For this review, take the finished solid that the model builds, in its own axes (mm). Face numbers are marked on the shaded views. A direction names the side the tool comes from. Round coordinates to 2 decimals unless told otherwise and drop trailing zeros. Order: outer loops, then holes, each group sorted by start corner. A loop starts at its lowest first (then second) coordinate and runs counter-clockwise, first axis right, second up. Notation, with made-up numbers: M 37,15 L 62,15 A30 cw 62,45 Z; hole C 56,13 d7. An arc over 180 degrees is marked long. Write item = value, one per line. Start each with the question number.
from build123d import *

# Parameters (mm, degrees)
SKETCH_1_R          = 7
SKETCH_1_R_2        = 3.45
EXTRUDE_1_DEPTH     = 10
SKETCH_2_R          = 8.05
SKETCH_2_R_2        = 4
CUT_EXTRUDE_1_DEPTH = 8


with BuildPart() as part:
    # 草图1 → 凸台-拉伸1 (new body)
    with BuildSketch(Plane.XY):
        Polygon((-25, 0), (25, 0), (25, 26), (13, 85), (-13, 85), (-25, 26), align=None)
        with Locations((0, 73)):
            Circle(SKETCH_1_R, mode=Mode.SUBTRACT)
        with Locations((-15, 13)):
            Circle(SKETCH_1_R_2, mode=Mode.SUBTRACT)
        with Locations((15, 13)):
            Circle(SKETCH_1_R_2, mode=Mode.SUBTRACT)
    extrude(amount=EXTRUDE_1_DEPTH)

    # 草图2 → 切除-拉伸1 (cut)
    with BuildSketch(Plane(origin=(0, 0, 0), x_dir=(-1, 0, 0), z_dir=(0, 0, -1))):
        with Locations((0, 73)):
            Circle(SKETCH_2_R)
        with Locations((0, 73)):
            Circle(SKETCH_2_R_2, mode=Mode.SUBTRACT)
    extrude(amount=-CUT_EXTRUDE_1_DEPTH, mode=Mode.SUBTRACT)


solid = part.part
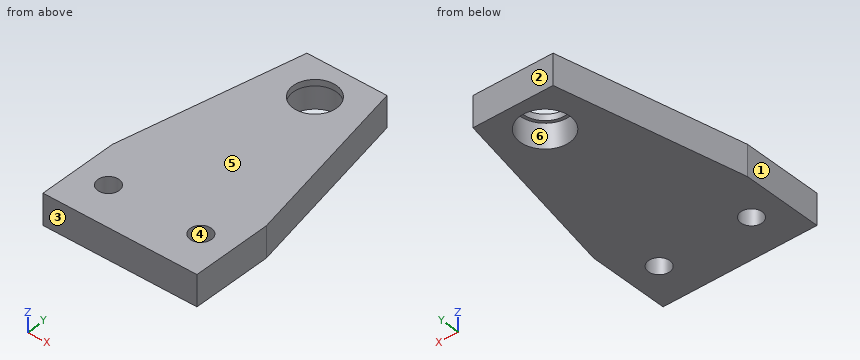
(1) We need section D-D, the plane y = 73. Write out the cut boundary in (x, z).
(2) We need section C-C, the plane z = 4.75. Write out the cut boundary in (x, y), then the cut area to 3 significant figures.
(3) For line 1 along Y through (x, z) = (0.5, 8.25); line 2 along Y through (x, z) = (0, 3); line 3 along X through (y, z) = (73, 9.1), list the stretches that pass through material, from the lowest coordinate up.
(4) We need section A-A, the plane x = 0. Write out the cut boundary in (y, z).
(5) We need section B-B, the plane y = 13. Write out the cut boundary in (x, z).
(6) Draft analysis for pull direction Y (two halves, no side actions). For the marked faces 1, 2, 3 and 4, state which applies: released by +Y, released by -Y, zero draft, split by the parting line, or undercut.
(7) Insertion check: pin 1 (1 mm diameter, centred on y = 51, z = 1, fed in from +X); pin 2 (4 mm diameter, centred on x = -15, y = 13, fed in from +Z); pin 3 (4 mm diameter, centred on y = 37, z = 5.5, fed in from +X); pin 4 (3 mm diameter, centred on y = 32.5, z = 5, fed in from +X). Each pin has a flat end and moves straight along its axis. Give the tip position at first contact, or say it passes through.
(8) For the marked faces 5 and 6, list the 3-axis set-ups (+Z, -Z, +X, -X, +Y, -Y) from which the entire face can be reached by the end or side of a thin tool; tool diameter is ignored.
Values:
q1.outline = M -15.44,0 L -8.05,0 L -8.05,8 L -7,8 L -7,10 L -15.44,10 Z; M 7,8 L 8.05,8 L 8.05,0 L 15.44,0 L 15.44,10 L 7,10 Z
q2.outline = M -25,0 L 25,0 L 25,26 L 13,85 L -13,85 L -25,26 Z; hole C -15,13 d6.9; hole C 0,73 d16.1; hole C 15,13 d6.9
q2.area = 3,260 mm²
q3.line_1 = 0 to 66.02, 79.98 to 85
q3.line_2 = 0 to 64.95, 81.05 to 85
q3.line_3 = -15.44 to -7, 7 to 15.44
q4.outline = M 0,0 L 64.95,0 L 64.95,8 L 66,8 L 66,10 L 0,10 Z; M 80,8 L 81.05,8 L 81.05,0 L 85,0 L 85,10 L 80,10 Z
q5.outline = M -25,0 L -18.45,0 L -18.45,10 L -25,10 Z; M -11.55,0 L 11.55,0 L 11.55,10 L -11.55,10 Z; M 18.45,0 L 25,0 L 25,10 L 18.45,10 Z
q6.face_1 = zero draft
q6.face_2 = released by +Y
q6.face_3 = released by -Y
q6.face_4 = undercut
q7.pin_1 = 20.02
q7.pin_2 = through
q7.pin_3 = 23.17
q7.pin_4 = 23.98
q8.face_5 = +Z, +X, -X, +Y, -Y
q8.face_6 = -Z
